from build123d import *

# Parameters (mm, degrees)
SKETCH3_W           = 10
SKETCH3_H           = 18
BOSS_EXTRUDE1_DEPTH = 3
BOSS_EXTRUDE2_DEPTH = 3
CUT_EXTRUDE1_DEPTH  = 4
SKETCH6_R           = 10
CUT_EXTRUDE2_DEPTH  = 4


with BuildPart() as part:
    # Sketch3 → Boss-Extrude1 (new body)
    with BuildSketch(Plane.XY):
        Polygon((0, 0), (56.979097759, 78.425), (-56.979097759, 78.425), align=None)
        with Locations((0, 68.425)):
            Rectangle(SKETCH3_W, SKETCH3_H, mode=Mode.SUBTRACT)
    extrude(amount=BOSS_EXTRUDE1_DEPTH)

    # Sketch4 → Boss-Extrude2 (add)
    with BuildSketch(Plane(origin=(0, 0, 0), x_dir=(-1, 0, 0), z_dir=(0, 0, -1))):
        Polygon((-56.979097759, 78.425), (-89.673511519, 123.425), (89.673511519, 123.425), (56.979097759, 78.425), align=None)
    extrude(amount=-BOSS_EXTRUDE2_DEPTH)

    # Sketch5 → Cut-Extrude1 (cut, through all)
    with BuildSketch(Plane.XY.offset(3)):
        Polygon((-89.673511519, 123.425), (-46.080959839, 123.425), (-67.877235679, 93.425), align=None)
        Polygon((89.673511519, 123.425), (46.080959839, 123.425), (67.877235679, 93.425), align=None)
    extrude(amount=-CUT_EXTRUDE1_DEPTH, mode=Mode.SUBTRACT)

    # Sketch6 → Cut-Extrude2 (cut, through all)
    with BuildSketch(Plane(origin=(0, 0, 0), x_dir=(-1, 0, 0), z_dir=(0, 0, -1))):
        Circle(SKETCH6_R)
    extrude(amount=-CUT_EXTRUDE2_DEPTH, mode=Mode.SUBTRACT)


solid = part.part
Source: CAD feature listing. Evaluate the final solid. Frame: model axes, mm. A direction names the side the tool comes from. Coordinates: 2 decimals unless noted, no trailing zeros. Loops run counter-clockwise (first coordinate to the right, second up) from the corner with the lowest first, then second, coordinate; pieces in that order, holes last. Notation, with made-up numbers: (-26.5, 20.25) -> (-0.5, 20.25) arc R35 ccw to (-0.5, 58.25) -> close; hole circle Ø5 at (88, 18.5). An arc over 180 degrees is marked (long way). Answer in a Markdown table with one row per item. Add a question column.
Q1. Section D-D on y = 22. Return the cut outline in (x, z).
Q2. Reachability of faces 1 (the face through (1, 123.425, 1)), 2 (the face through (0, 77.425, 1)) from +Z, -Z, +X, -X, +Y, -Y: full face, straight path, thin tool, end or side. Return the list, or none.
Q3. Section A-A on z = 1.4. Return the cut outline in (x, y) (3 decimals).
Q4. Section B-B on y = 62.5. Return the cut outline in (x, z), and give its area (3 significant figures).
Q5. Contact query for flat-ended pins moving along their axis: pin 1 Ø1.5 at (y, z) = (88, 1.5) entering from -X; pin 2 Ø0.9 at (x, z) = (1.5, 1.5) entering from -Y; pin 3 Ø1.5 at (y, z) = (74.5, 2) entering from -X. Output: stop coordinate, or through.
Q6. Pull-direction query (X, two-part tool) for faces 3 (the face through (0, 10, 1)), 4 (the face through (-1, 79, 3)), 5 (the face through (56.827, 108.635, 1.521)); classes: pulls with the +X half, pulls with the -X half, needs draft (parallel to the pull), parting line crosses it, or undercut.
Q7. Ray query, line 1 along X through (y, z) = (75.5, 0.55); line 2 along X through (y, z) = (65.5, 1.25); line 3 along Y through (x, z) = (-3.5, 2.4) (1 decimal). Return the intervals inside material, ascending.
Q8. Section C-C on x = -34. Return the cut outline in (y, z) (3 decimals), and give its area (3 significant figures).
Computed values:
| question | item | result |
|---|---|---|
| 1 | outline | (-15.98, 0) -> (15.98, 0) -> (15.98, 3) -> (-15.98, 3) -> close |
| 2 | face 1 | +Z, -Z, +X, -X, +Y |
| 2 | face 2 | +Z, -Z |
| 3 | outline | (-67.877, 93.425) -> (-5.878, 8.09) arc R10 cw to (5.878, 8.09) -> (67.877, 93.425) -> (46.081, 123.425) -> (-46.081, 123.425) -> close; hole (-5, 59.425) -> (5, 59.425) -> (5, 77.425) -> (-5, 77.425) -> close |
| 4 | outline | (-45.41, 0) -> (-5, 0) -> (-5, 3) -> (-45.41, 3) -> close; (5, 0) -> (45.41, 0) -> (45.41, 3) -> (5, 3) -> close |
| 4 | area | 242 mm^2 |
| 5 | pin 1 | stops at x = -64.48 |
| 5 | pin 2 | stops at y = 9.81 |
| 5 | pin 3 | stops at x = -54.67 |
| 6 | face 3 | undercut |
| 6 | face 4 | needs draft |
| 6 | face 5 | pulls with the +X half |
| 7 | line 1 | x = -54.85 to -5, 5 to 54.85 |
| 7 | line 2 | x = -47.59 to -5, 5 to 47.59 |
| 7 | line 3 | y = 9.4 to 59.4, 77.4 to 123.4 |
| 8 | outline | (46.797, 0) -> (123.425, 0) -> (123.425, 3) -> (46.797, 3) -> close |
| 8 | area | 230 mm^2 |
